CAD build for the part. Positions are in the model's coordinates, mm. Face numbers are marked on the shaded views. A direction names the side the tool comes from. Give positions to 0.01 mm unless a question says otherwise; leave off trailing zeros. Order: outer loops, then holes, each group sorted by start corner. A loop starts at its lowest first (then second) coordinate and runs counter-clockwise, first axis right, second up.
Item 1: Which spindle directions (+Z, -Z, +X, -X, +Y, -Y) get a long thin tool onto all of the face, cutting with end or side? Do the marked faces 1 and 2. Say none if no direction does.
Item 2: Flat gauge pins, fed straight in: P1, Ø2.5, axis at x = 25.5, y = 17, coming from the +Z side; P2, Ø6.5, axis at x = 26.12, y = 15.08, coming from the -Z side; P3, Ø6, axis at y = -12.5, z = 37.5, coming from the -X side; P4, Ø3, axis at x = -12.5, z = 14, coming from the +Y side. Where does each tip first touch, or does it go through?
Item 3: Wall check: L1, parallel to Y at x = 0, z = 48; L2, parallel to Z at x = 29, y = -9; L3, parallel to Y at x = -0.5, z = 22. Give the ranges that are in metal, low to high.
Item 4: Band-saw the part on B-B on x = 0. Count the separate pieces of the cut face and the enclosed holes in it, plus the area to 3 significant figures.
Item 5: Band-saw the part on A-A on y = 0. Give the cut face in (x, z) (3 decimals), plus the area to 3 significant figures.
Item 6: Band-saw the part on D-D on z = 31.5. Give the cut face in (x, y), plus the area to 3 significant figures.
Item 7: Two-plate mould, pull along Y, no slides. Class the marked faces 3, 4 and 5: released by +Y, released by -Y, zero draft, split by the parting line, or undercut.
Item 8: Band-saw the part on C-C on z = 8.5. Give the cut face in (x, y).
Autodesk Fusion 360 part; units mm, degrees
sketch "Sketch1" plane through (0, 0, 0) normal (0, 0, 1) x (1, 0, 0)
  circle A0 centre (0, 0) radius 16.51
  circle A1 centre (0, 0) radius 12.7
  circle A2 centre (0, 0) radius 38.1
  dimension "d1" = 33.02
  dimension "d2" = 25.4
  dimension "d3" = 76.2
extrude "Extrude1" add sketch "Sketch1" along normal blind 50.8 contours A0
extrude "Extrude2" add sketch "Sketch1" against normal blind 4.572 contours A0 | A2
sketch "Sketch3" plane through (0, 0, 0) normal (0, 0, 1) x (1, 0, 0)
  line L0 (0, 0) -> (0, -39.9504) construction
  line L1 (0, 0) -> (-48.5556, 28.0336) construction
  line L2 (0, 0) -> (38.9341, 22.4786) construction
  circle A0 centre (0, 0) radius 30.1625 construction
  circle A1 centre (0, -30.1625) radius 2.159
  circle A2 centre (-26.1215, 15.0812) radius 2.159
  circle A3 centre (26.1215, 15.0812) radius 2.159
  circle A4 centre (0, -30.1625) radius 4.191
  circle A5 centre (-26.1215, 15.0812) radius 4.191
  circle A6 centre (26.1215, 15.0812) radius 4.191
  dimension "d8" = 120
  dimension "d9" = 120
  dimension "d10" = 60.325
  dimension "d11" = 4.318
  dimension "d12" = 8.382
extrude "Extrude3" cut sketch "Sketch3" against normal up to surface (4.572 mm away) contours A1 | A2 | A3
extrude "Extrude4" cut sketch "Sketch3" against normal blind 1.5875
sketch "Sketch4" plane through (0, 0, 0) normal (0, 1, 0) x (1, 0, 0)
  line L0 (0, 0) -> (0, -68.6315) construction
  circle A0 centre (0, -38.1) radius 3.1
  line L1 (0, 0) -> (-36.56, 0) construction
  line L2 (-16.51, -50.8) -> (16.51, -50.8) construction
  dimension "d17" = 6.2
  dimension "d19" = 12.7
extrude "Extrude5" cut sketch "Sketch4" against normal blind 28.9814
sketch "Sketch5" plane through (0, 0, 0) normal (0, 0, 1) x (-1, 0, 0)
  circle A0 centre (-26.1215, -15.0812) radius 4.191
  circle A1 centre (26.1215, -15.0812) radius 4.191
  circle A2 centre (0, 30.1625) radius 4.191
  circle A3 centre (0, 0) radius 38.1
  circle A4 centre (0, 0) radius 16.51
  circle A5 centre (0, 0) radius 16.51
  circle A6 centre (0, 0) radius 20.574
  dimension "d22" = 41.148
extrude "Extrude6" add sketch "Sketch5" along normal blind 28.575 contours A6
fillet "Fillet1" radius 3.81 1 edges at (19.1817, -7.4399, 0)
fillet "Fillet2" radius 1.27 1 edges at (-35.5217, -13.7775, 0)
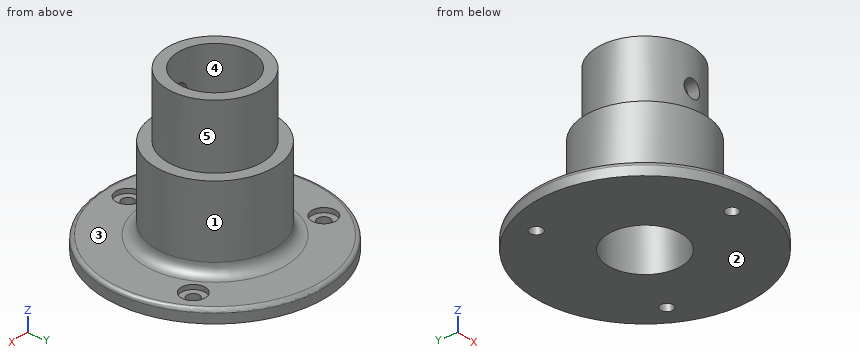
The answers:
1. face 1: +Z
1. face 2: -Z, +X, -X, +Y, -Y
2. P1: stops at z = -1.59
2. P2: stops at z = -4.57
2. P3: stops at x = -13.5
2. P4: stops at y = 17.39
3. L1: y = -16.51 to -12.7, 12.7 to 16.51
3. L2: z = -4.57 to 0
3. L3: y = -20.57 to -12.69, 12.69 to 20.57
4. separate pieces: 4
4. enclosed holes: 0
4. area: 807 mm2
5. outline: (-38.1, -4.572) - (-12.7, -4.572) - (-12.7, 50.8) - (-16.51, 50.8) - (-16.51, 28.575) - (-20.574, 28.575) - (-20.574, 3.81) arc R3.81 cw to (-24.384, 0) - (-36.83, 0) arc R1.27 ccw to (-38.1, -1.27) - close; (12.7, -4.572) - (38.1, -4.572) - (38.1, -1.27) arc R1.27 ccw to (36.83, 0) - (24.384, 0) arc R3.81 cw to (20.574, 3.81) - (20.574, 28.575) - (16.51, 28.575) - (16.51, 50.8) - (12.7, 50.8) - close
5. area: 857 mm2
6. outline: circle Ø33.02 at (0, 0); hole circle Ø25.4 at (0, 0)
6. area: 350 mm2
7. face 3: zero draft
7. face 4: undercut
7. face 5: split by the parting line
8. outline: circle Ø41.15 at (0, 0); hole circle Ø25.4 at (0, 0)
